Autodesk Inventor part; units mm, degrees
ref_plane "YZ Plane" through (0, 0, 0) normal (1, 0, 0) x (0, 1, 0)
ref_plane "XZ Plane" through (0, 0, 0) normal (0, 1, 0) x (-1, 0, 0)
ref_plane "XY Plane" through (0, 0, 0) normal (0, 0, 1) x (1, 0, 0)
sketch "Sketch1" plane through (0, 0, 0) normal (0, 0, 1) x (1, 0, 0)
  line L0 (0, 0) -> (-150, 0)
  line L1 (-150, 0) -> (-150, 95)
  line L2 (-150, 95) -> (0, 95)
  line L3 (0, 95) -> (0, 0)
  dimension "d0" = 150
  dimension "d1" = 95
extrude "Extrusion1" add sketch "Sketch1" along normal blind 15
sketch "Sketch2" plane through (0, 0, 15) normal (0, 0, 1) x (1, 0, 0)
  line L0 (-32.5, 5) -> (-117.5, 5)
  line L1 (-117.5, 5) -> (-117.5, 90)
  line L2 (-117.5, 90) -> (-32.5, 90)
  line L3 (-32.5, 90) -> (-32.5, 5)
  point P0 (0, 0)
  dimension "d4" = 85
  dimension "d5" = 85
extrude "Extrusion2" cut sketch "Sketch2" against normal blind 2
sketch "Sketch3" plane through (0, 0, 13) normal (0, 0, 1) x (1, 0, 0)
  line L0 (-47.5, 75) -> (-102.5, 75)
  line L1 (-102.5, 75) -> (-102.5, 20)
  line L2 (-102.5, 20) -> (-47.5, 20)
  line L3 (-47.5, 20) -> (-47.5, 75)
  point P0 (0, 0)
  point P1 (-47.5, 47.5)
  dimension "d10" = 55
  dimension "d11" = 55
extrude "Extrusion3" cut sketch "Sketch3" against normal blind 2
sketch "Sketch4" plane through (0, 0, 0) normal (0, 0, -1) x (-1, 0, 0)
  circle A0 centre (75, 47.5) radius 14.25
  circle A1 centre (75, 47.5) radius 17.15
  line L0 (2.5, 2.5) -> (7.5, 2.5)
  line L1 (7.5, 2.5) -> (7.5, 7.5)
  line L2 (7.5, 7.5) -> (2.5, 7.5)
  line L3 (2.5, 7.5) -> (2.5, 2.5)
  line L4 (147.5, 2.5) -> (142.5, 2.5)
  line L5 (142.5, 2.5) -> (142.5, 7.5)
  line L6 (142.5, 7.5) -> (147.5, 7.5)
  line L7 (147.5, 7.5) -> (147.5, 2.5)
  line L8 (2.5, 92.5) -> (7.5, 92.5)
  line L9 (7.5, 92.5) -> (7.5, 87.5)
  line L10 (7.5, 87.5) -> (2.5, 87.5)
  line L11 (2.5, 87.5) -> (2.5, 92.5)
  line L12 (147.5, 92.5) -> (142.5, 92.5)
  line L13 (142.5, 92.5) -> (142.5, 87.5)
  line L14 (142.5, 87.5) -> (147.5, 87.5)
  line L15 (147.5, 87.5) -> (147.5, 92.5)
  point P0 (0, 0)
  dimension "d14" = 28.5
  dimension "d15" = 34.3
  dimension "d16" = 5
  dimension "d17" = 5
  dimension "d18" = 5
  dimension "d19" = 5
  dimension "d20" = 5
  dimension "d21" = 5
  dimension "d22" = 5
  dimension "d23" = 5
extrude "Extrusion4" cut sketch "Sketch4" against normal blind 5
properties part number "Shoulder_Both_Marker_V1"
Here's how the part is built. I have some questions about the finished solid (model axes, mm). A direction names the side the tool comes from. Give positions to 0.01 mm unless a question says otherwise; leave off trailing zeros. Order: outer loops, then holes, each group sorted by start corner. A loop starts at its lowest first (then second) coordinate and runs counter-clockwise, first axis right, second up. Notation, with made-up numbers: (14, 12.5) -> (57, 12.5) arc R7 cw to (57, 17.5) -> close; hole circle Ø10 at (84.5, 37). An arc over 180 degrees is marked (long way). One line per item, written item: value. Start each with the question number.
1. Imagine slicing it at C-C, the plane x = -109.5. List the corners of the cut face in (y, z) for me.
2. Imagine slicing it at B-B, the plane y = 12.5. List the corners of the cut face in (x, z) for me, plus the area to 3 significant figures.
3. For faces 4 (the face through (-142.5, 5, 2)), 5 (the face through (-150, 47, 7)), 6 (the face through (-75, 48, 11)), which set-ups out of +Z, -Z, +X, -X, +Y, -Y let a thin tool reach every point of the face, with its end or its side?
4. Imagine slicing it at D-D, the plane y = 23. List the corners of the cut face in (x, z) for me, plus the area to 3 significant figures.
5. We'd pull the mould along Y, two halves only. Please class faces 1 (the face through (-75, 48, 0)), 2 (the face through (-76, 95, 7)), 3 (the face through (-7.5, 90, 2)): released by +Y, released by -Y, zero draft, split by the parting line, or undercut.
6. Imagine slicing it at A-A, the plane z = 2.75. List the corners of the cut face in (x, y) for me, plus the area to 3 significant figures.
7. Will these pins go through, and if not, where does the flat tip stop? pin 1 Ø4 at (x, y) = (-114.5, 75.5) entering from +Z; pin 2 Ø4 at (x, y) = (-6, 91) entering from -Z; pin 3 Ø2.5 at (x, y) = (-144.5, 4) entering from -Z.
8. I need wall thicknesses on probe 1 along Y at (x, z) = (-75, 1.75); probe 2 along X at (y, z) = (4.5, 1); probe 3 along X at (y, z) = (38, 12). Which ranges of each line are inside material? Lowest first, please. Write a range as from..to.
Values follow:
1. outline: (0, 0) -> (95, 0) -> (95, 15) -> (90, 15) -> (90, 13) -> (5, 13) -> (5, 15) -> (0, 15) -> close
2. outline: (-150, 0) -> (0, 0) -> (0, 15) -> (-32.5, 15) -> (-32.5, 13) -> (-117.5, 13) -> (-117.5, 15) -> (-150, 15) -> close
2. area: 2,080 mm2
3. face 4: -Z
3. face 5: +Z, -Z, -X, +Y, -Y
3. face 6: +Z
4. outline: (-150, 0) -> (0, 0) -> (0, 15) -> (-32.5, 15) -> (-32.5, 13) -> (-47.5, 13) -> (-47.5, 11) -> (-102.5, 11) -> (-102.5, 13) -> (-117.5, 13) -> (-117.5, 15) -> (-150, 15) -> close
4. area: 1,970 mm2
5. face 1: zero draft
5. face 2: released by +Y
5. face 3: undercut
6. outline: (-150, 0) -> (0, 0) -> (0, 95) -> (-150, 95) -> close; circle Ø28.5 at (-75, 47.5); hole (-147.5, 2.5) -> (-142.5, 2.5) -> (-142.5, 7.5) -> (-147.5, 7.5) -> close; hole (-147.5, 87.5) -> (-142.5, 87.5) -> (-142.5, 92.5) -> (-147.5, 92.5) -> close; hole circle Ø34.3 at (-75, 47.5); hole (-7.5, 2.5) -> (-2.5, 2.5) -> (-2.5, 7.5) -> (-7.5, 7.5) -> close; hole (-7.5, 87.5) -> (-2.5, 87.5) -> (-2.5, 92.5) -> (-7.5, 92.5) -> close
6. area: 13,900 mm2
7. pin 1: stops at z = 13
7. pin 2: stops at z = 0
7. pin 3: stops at z = 5
8. probe 1: y = 0..30.35, 33.25..61.75, 64.65..95
8. probe 2: x = -150..-147.5, -142.5..-7.5, -2.5..0
8. probe 3: x = -150..-102.5, -47.5..0
